Study the drawing (mm; zero at the part's minimum x, y, z) and answer. A direction names the side the tool comes from. Coordinates: 2 decimals unless noted, no trailing zeros. Order: outer loops, then holes, each group sorted by start corner. A loop starts at its lowest first (then second) coordinate and runs counter-clockwise, first axis right, second up. Notation, with made-up numbers: M -34.75,24.25 L 22.25,24.25 A11 ccw 22.25,35.25 Z; hole C 55,-8.5 d3. An arc over 180 degrees is marked long. Put each result on its own line as item: value.
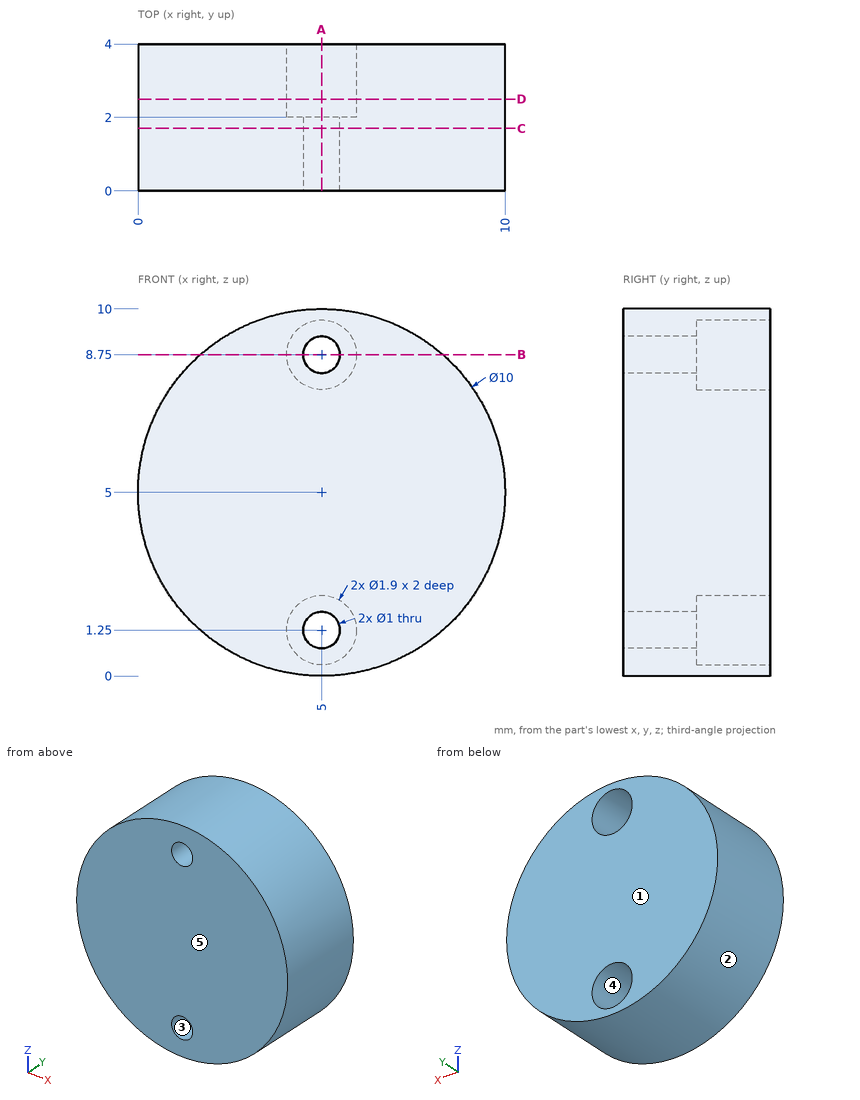
Q1. For a pull along Z with two mould halves and no side action, classify the marked faces 1, 2 and 3 as +Z half, -Z half, draft (parallel to the pull), parting line (faces both ways), or undercut.
Answers below:
face 1: draft
face 2: parting line
face 3: undercut
Q2. Find section A-A on x = 5. Write down the section's boundary in (y, z).
Answers below:
outline: M 0,0 L 4,0 L 4,0.3 L 2,0.3 L 2,0.75 L 0,0.75 Z; M 0,1.75 L 2,1.75 L 2,2.2 L 4,2.2 L 4,7.8 L 2,7.8 L 2,8.25 L 0,8.25 Z; M 0,9.25 L 2,9.25 L 2,9.7 L 4,9.7 L 4,10 L 0,10 Z
Q3. A tool of negligible diameter and unlimited length cuts with its end or side. For the marked faces 4 and 5, from which of +Z, -Z, +X, -X, +Y, -Y can it reach the whole face along a straight path? Write none if from no direction.
Answers below:
face 4: +Y
face 5: +Z, -Z, +X, -X, -Y
Q4. Given pin 1 (2 mm diameter, centred on y = 2.5, z = 2, fed in from -X); pin 2 (1.5 mm diameter, centred on x = 7.5, y = 3, fed in from +Z); pin 3 (1.5 mm diameter, centred on y = 0.5, z = 6.5, fed in from +X), each flat-ended and moving along its own axis, determine where each tip first touches the part or whether it passes through.
Answers below:
pin 1: stops at x = 0.42
pin 2: stops at z = 9.68
pin 3: stops at x = 9.94
Q5. Find section D-D on y = 2.5. Write down the section's boundary in (x, z), plus the area to 3 significant figures.
Answers below:
outline: C 5,5 d10; hole C 5,1.25 d1.9; hole C 5,8.75 d1.9
area: 72.9 mm^2
Q6. Find section B-B on z = 8.75. Write down the section's boundary in (x, y).
Answers below:
outline: M 1.69,0 L 4.5,0 L 4.5,2 L 4.05,2 L 4.05,4 L 1.69,4 Z; M 5.5,0 L 8.31,0 L 8.31,4 L 5.95,4 L 5.95,2 L 5.5,2 Z
Q7. Consider line 1 along Z through (x, y) = (5, 1.2); line 2 along Z through (x, y) = (5, 2.95); line 3 along X through (y, z) = (3, 1.25). Determine where each line is inside the solid, lowest interval first.
Answers below:
line 1: z = 0 to 0.75, 1.75 to 8.25, 9.25 to 10
line 2: z = 0 to 0.3, 2.2 to 7.8, 9.7 to 10
line 3: x = 1.69 to 4.05, 5.95 to 8.31
Q8. Find section C-C on y = 1.7. Write down the section's boundary in (x, z), plus the area to 3 significant figures.
Answers below:
outline: C 5,5 d10; hole C 5,1.25 d1; hole C 5,8.75 d1
area: 77.0 mm^2
